Geometry check sheet. Reference: the model listing, model coordinates, mm. A direction names the side the tool comes from. Round coordinates to 2 decimals unless told otherwise and drop trailing zeros. Order: outer loops, then holes, each group sorted by start corner. A loop starts at its lowest first (then second) coordinate and runs counter-clockwise, first axis right, second up. Notation, with made-up numbers: M 22,57 L 58,57 A24 ccw 58,88 Z; hole C 56,59.5 d11. An arc over 180 degrees is marked long. Return JSON: item names as keys, results as strings. Group by question number.
```python
from build123d import *

# Parameters (mm, degrees)
BOSS_EXTRUDE1_DEPTH          = 5.08
P_0_323_DIAMETER_HOLE1_D     = 8.2042
P_0_323_DIAMETER_HOLE1_DEPTH = 16.51
P_0_323_DIAMETER_HOLE1_TIP   = 2.464790345


with BuildPart() as part:
    # Sketch1 → Boss-Extrude1 (new body)
    with BuildSketch(Plane(origin=(0, 0, 0), x_dir=(1, 0, 0), z_dir=(0, 1, 0))):
        Polygon((-16.1925, 0), (16.1925, 0), (16.1925, 7.62), (11.1125, 7.62), (11.1125, 68.58), (16.1925, 68.58), (16.1925, 76.2), (-16.1925, 76.2), (-16.1925, 68.58), (-11.1125, 68.58), (-11.1125, 7.62), (-16.1925, 7.62), align=None)
    extrude(amount=BOSS_EXTRUDE1_DEPTH)

    # P (0.323) Diameter Hole1
    with Locations(Plane(origin=(0, 5.08, 0), x_dir=(1, 0, 0), z_dir=(0, 1, 0))):
        with Locations((0, 57.15), (0, 19.05)):
            Hole(P_0_323_DIAMETER_HOLE1_D / 2, depth=P_0_323_DIAMETER_HOLE1_DEPTH)
            with Locations((0, 0, -(P_0_323_DIAMETER_HOLE1_DEPTH + P_0_323_DIAMETER_HOLE1_TIP / 2))):  # 118° drill point
                Cone(0, P_0_323_DIAMETER_HOLE1_D / 2, P_0_323_DIAMETER_HOLE1_TIP, mode=Mode.SUBTRACT)


solid = part.part
```
Q1. Material ranges on line 1 along Z through (x, y) = (0, 3.3); line 2 along X through (y, z) = (2.3, -19.05); line 3 along X through (y, z) = (0.35, -8.5), recorded low to high.
Q2. Set-up check for faces 1 (the face through (14, 3, -68.58)), 2 (the face through (-14, 3, -7.62)), 3 (the face through (16.192, 3, -72)): record each of +Z, -Z, +X, -X, +Y, -Y from which the full face is reachable in a straight line by a thin tool's end or side.
Q3. Section check B-B on x = 0. Record the cut outline in (y, z), plus the area to 3 significant figures.
Q4. Section check C-C on y = 1.05. Record the cut outline in (x, z).
Q5. Section check A-A on z = -19.05. Record the cut outline in (x, y), plus the area to 3 significant figures.
Q6. Section check D-D on z = -51. Record the cut outline in (x, y).
Q7. Depth check by flat-ended pin: pin 1 Ø2.5 at (y, z) = (2, -23.5) entering from -X. Enter the tip coordinate at first touch or a pass-through.
Geometry check:
{
 "1": {"line 1": "z = -76.2 to -61.25, -53.05 to -23.15, -14.95 to 0", "line 2": "x = -11.11 to -4.1, 4.1 to 11.11", "line 3": "x = -11.11 to 11.11"},
 "2": {"face 1": "+X, +Y, -Y", "face 2": "-X, +Y, -Y", "face 3": "+Z, -Z, +X, +Y, -Y"},
 "3": {"outline": "M 0,-76.2 L 5.08,-76.2 L 5.08,-61.25 L 0,-61.25 Z; M 0,-53.05 L 5.08,-53.05 L 5.08,-23.15 L 0,-23.15 Z; M 0,-14.95 L 5.08,-14.95 L 5.08,0 L 0,0 Z", "area": "304 mm^2"},
 "4": {"outline": "M -16.19,-76.2 L 16.19,-76.2 L 16.19,-68.58 L 11.11,-68.58 L 11.11,-7.62 L 16.19,-7.62 L 16.19,0 L -16.19,0 L -16.19,-7.62 L -11.11,-7.62 L -11.11,-68.58 L -16.19,-68.58 Z; hole C 0,-57.15 d8.2; hole C 0,-19.05 d8.2"},
 "5": {"outline": "M -11.11,0 L -4.1,0 L -4.1,5.08 L -11.11,5.08 Z; M 4.1,0 L 11.11,0 L 11.11,5.08 L 4.1,5.08 Z", "area": "71.2 mm^2"},
 "6": {"outline": "M -11.11,0 L 11.11,0 L 11.11,5.08 L -11.11,5.08 Z"},
 "7": {"pin 1": "stops at x = -11.11"}
}
